from build123d import *

# Parameters (mm, degrees)
SKETCH12_W                = 50
SKETCH12_H                = 12.7
BOSS_EXTRUDE1_DEPTH       = 112
M5X0_8_TAPPED_HOLE2_D     = 4.2
M5X0_8_TAPPED_HOLE2_DEPTH = 14.4
M5X0_8_TAPPED_HOLE2_TIP   = 1.2618073
M5X0_8_TAPPED_HOLE3_D     = 4.2
SKETCH19_W                = 34
SKETCH19_H                = 52.9
CUT_EXTRUDE1_DEPTH        = 9.7
FILLET1_R                 = 5


with BuildPart() as part:
    # Sketch12 → Boss-Extrude1 (new body)
    with BuildSketch(Plane.XY):
        Rectangle(SKETCH12_W, SKETCH12_H)
    extrude(amount=BOSS_EXTRUDE1_DEPTH)

    # M5x0.8 Tapped Hole2
    with Locations(Plane(origin=(0, 0, 0), x_dir=(-1, 0, 0), z_dir=(0, 0, -1))):
        with Locations((-17.5, 0), (0, 0), (17.5, 0)):
            Hole(M5X0_8_TAPPED_HOLE2_D / 2, depth=M5X0_8_TAPPED_HOLE2_DEPTH)
            with Locations((0, 0, -(M5X0_8_TAPPED_HOLE2_DEPTH + M5X0_8_TAPPED_HOLE2_TIP / 2))):  # 118° drill point
                Cone(0, M5X0_8_TAPPED_HOLE2_D / 2, M5X0_8_TAPPED_HOLE2_TIP, mode=Mode.SUBTRACT)

    # M5x0.8 Tapped Hole3 (through all)
    with Locations(Plane(origin=(0, 6.35, 0), x_dir=(1, 0, 0), z_dir=(0, 1, 0))):
        with Locations((-0.5, -37.3), (15.5, -37.3), (15.5, -106.2), (-0.5, -106.2)):
            Hole(M5X0_8_TAPPED_HOLE3_D / 2)

    # Sketch19 → Cut-Extrude1 (cut)
    with BuildSketch(Plane(origin=(0, -6.35, 0), x_dir=(1, 0, 0), z_dir=(0, 1, 0))):
        with Locations((0, -71.75)):
            Rectangle(SKETCH19_W, SKETCH19_H)
    extrude(amount=CUT_EXTRUDE1_DEPTH, mode=Mode.SUBTRACT)

    # Fillet1
    fillet1_edges = [part.edges().sort_by_distance(p)[0] for p in [
        (-25, 0, 112),
        (25, 0, 112),
        (-17, -1.5, 45.3),
        (-17, -1.5, 98.2),
        (17, -1.5, 98.2),
        (17, -1.5, 45.3),
    ]]
    fillet(fillet1_edges, radius=FILLET1_R)


solid = part.part
Could you check a few things on this model? Use its own coordinates, in mm. A direction names the side the tool comes from. Give positions to 0.01 mm unless a question says otherwise; leave off trailing zeros. Loops run counter-clockwise (first coordinate to the right, second up) from the corner with the lowest first, then second, coordinate; pieces in that order, holes last. Notation, with made-up numbers: M 35.5,-4 L 62.5,-4 A17 cw 62.5,7 Z; hole C 67,77 d2. An arc over 180 degrees is marked long. Answer as a JSON object with one key per item and string values.
Q1. Suppose I cut it at D-D, the plane z = 12. List the corners of the cut face in (x, y) for me.
Values found:
{"outline": "M -25,-6.35 L 25,-6.35 L 25,6.35 L -25,6.35 Z; hole C -17.5,0 d4.2; hole C 0,0 d4.2; hole C 17.5,0 d4.2"}
Q2. Suppose I cut it at B-B, the plane x = -7.5. List the corners of the cut face in (y, z) for me, plus the area to 3 significant figures.
Values found:
{"outline": "M -6.35,0 L 6.35,0 L 6.35,112 L -6.35,112 L -6.35,98.2 L 3.35,98.2 L 3.35,45.3 L -6.35,45.3 Z", "area": "909 mm²"}
Q3. Suppose I cut it at A-A, the plane z = 37.3. List the corners of the cut face in (x, y) for me, plus the area to 3 significant figures.
Values found:
{"outline": "M -25,-6.35 L -2.6,-6.35 L -2.6,6.35 L -25,6.35 Z; M 1.6,-6.35 L 13.4,-6.35 L 13.4,6.35 L 1.6,6.35 Z; M 17.6,-6.35 L 25,-6.35 L 25,6.35 L 17.6,6.35 Z", "area": "528 mm²"}
Q4. Suppose I cut it at C-C, the plane y = -3.5. List the corners of the cut face in (x, z) for me.
Values found:
{"outline": "M -25,0 L 25,0 L 25,107 A5 ccw 20,112 L -20,112 A5 ccw -25,107 Z; hole M -17,50.3 A5 ccw -12,45.3 L 12,45.3 A5 ccw 17,50.3 L 17,93.2 A5 ccw 12,98.2 L -12,98.2 A5 ccw -17,93.2 Z; hole C -0.5,37.3 d4.2; hole C -0.5,106.2 d4.2; hole C 15.5,37.3 d4.2; hole C 15.5,106.2 d4.2"}
Q5. For P1, Ø2, axis at x = -0.5, y = 3, coming from the -Z side; P2, Ø3.5, axis at x = 15.5, z = 106.2, coming from the -Y side (3 decimals); P3, Ø12, axis at x = -4.5, z = 62, coming from the -Y side, each with a flat end and sliding along its axis, tell me the tip position at first contact or that it passes through.
Values found:
{"P1": "stops at z = 0", "P2": "passes through", "P3": "stops at y = 3.35"}
Q6. If we mould it in two halves opening along Z, with no side actions, what happens to faces 1 (the cylindrical face through (2.003, 0.631, 7.301)), 2 (the flat face through (0, -3, 0)), 3 (the flat face through (0, 3.35, 71))? For each: pulls with the +Z half, pulls with the -Z half, needs draft (parallel to the pull), parting line crosses it, or undercut.
Values found:
{"face 1": "needs draft", "face 2": "pulls with the -Z half", "face 3": "undercut"}
Q7. If I drill on probe 1 along X at (y, z) = (2.75, 106.2); probe 2 along Z at (x, y) = (15.5, 3); probe 3 along Z at (x, y) = (-11, 0.5), over which ranges is the centre line in solid material (lowest first)? Write a range as [from, to].
Values found:
{"probe 1": "x = [-25, -2.6], [1.6, 13.4], [17.6, 25]", "probe 2": "z = [0, 35.2], [39.4, 46.73], [96.77, 104.1], [108.3, 112]", "probe 3": "z = [0, 45.3], [98.2, 112]"}
Q8. For faces 4 (the flat face through (0, 6.35, 55)), 5 (the cylindrical face through (-15.497, 0.631, 7.301)), 6 (the cylindrical face through (-15.5, -1.43, 96.77)), which set-ups out of +Z, -Z, +X, -X, +Y, -Y let a thin tool reach every point of the face, with its end or its side?
Values found:
{"face 4": "+Z, -Z, +X, -X, +Y", "face 5": "-Z", "face 6": "-Y"}
